Source: CAD feature listing. Evaluate the final solid. Frame: model axes, mm. Face numbers are marked on the shaded views. Give positions to 0.01 mm unless a question says otherwise; leave off trailing zeros. Order: outer loops, then holes, each group sorted by start corner. A loop starts at its lowest first (then second) coordinate and runs counter-clockwise, first axis right, second up.
1) Draft query along X for the marked faces 1, 2 and 3. Return one class per face: released by +X, released by -X, zero draft, split by the parting line, or undercut.
2) First-contact query: P1, Ø3, axis at x = -108.5, y = 10.5, coming from the -Z side; P2, Ø5, axis at x = -142, z = 5, coming from the +Y side. Flat tips, straight axial feed; report the tip coordinate or a pass-through.
3) Material intervals for line 1 (X direction, y = 13.5, z = -7.75); line 2 (X direction, y = 14.75, z = 5.5); line 3 (Z direction, x = 1.35, y = 10), sorted ascending.
4) Section A-A, the plane x = -133. Return loops of the section in (y, z), plus the area to 3 significant figures.
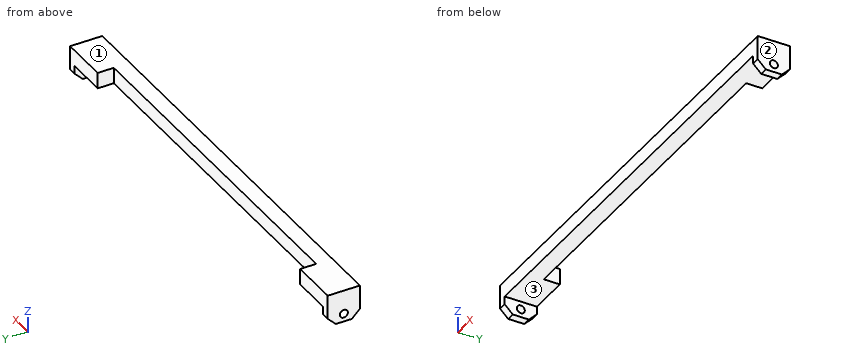
Autodesk Fusion 360 part; units mm, degrees
sketch "Sketch1" plane through (0, 0, 0) normal (0, 1, 0) x (1, 0, 0)
  line L0 (0, 0) -> (-25, 0)
  line L1 (-25, 0) -> (-25, -5)
  line L2 (-25, -5) -> (5, -5)
  line L3 (0, 0) -> (0, 10)
  line L4 (0, 10) -> (5, 10)
  line L5 (5, 10) -> (5, -5)
  line L6 (-25, 0) -> (-245, 0)
  line L7 (-245, 0) -> (-245, -5)
  line L8 (-245, -5) -> (-25, -5)
  line L9 (-25, 0) -> (-140, 0)
  line L10 (-140, 0) -> (-140, 27.0089)
  line L11 (-270, 10) -> (-275, 10)
  line L12 (-270, 0) -> (-270, 10)
  line L13 (-275, 10) -> (-275, -5)
  line L14 (-270, 0) -> (-245, 0)
  line L15 (-245, -5) -> (-275, -5)
  line L16 (-245, 0) -> (-245, -5)
  point P0 (-270, 0)
  dimension "d1" = 25
  dimension "d2" = 5
  dimension "d3" = 30
  dimension "d4" = 10
  dimension "d5" = 5
  dimension "d6" = 220
  dimension "d7" = 5
  dimension "d8" = 115
extrude "Extrude1" add sketch "Sketch1" along normal blind 10
extrude "Extrude2" add sketch "Sketch1" along normal blind 20 contours L0 L1 L2 L3 L4 L5 | L7 L11 L12 L13 L14 L15 L16
sketch "Sketch2" plane through (5, 0, 0) normal (1, 0, 0) x (0, 0, -1)
  line L0 (-5, 0) -> (10, 0)
  line L1 (10, 0) -> (10, 20)
  line L2 (10, 20) -> (-5, 20)
  line L3 (-5, 20) -> (-5, 0)
sketch "Sketch3" plane through (0, 0, 0) normal (-1, 0, 0) x (0, 0, 1)
  line L0 (-10, 0) -> (0, 0)
  line L1 (0, 0) -> (0, 20)
  line L2 (0, 20) -> (-10, 20)
  line L3 (-10, 20) -> (-10, 0)
  line L4 (-10, 0) -> (-5, 0)
  line L5 (-5, 0) -> (-5, 10)
  circle A0 centre (-5, 10) radius 2.5
  dimension "d13" = 5
  dimension "d14" = 10
  dimension "d15" = 5
extrude "Extrude3" cut sketch "Sketch3" along normal mid plane 662 contours A0
chamfer "Chamfer1" distance 5 angle 45 4 edges at (2.5, 20, -10) (2.5, 0, -10) (-272.5, 20, -10) (-272.5, 0, -10)
sketch "Sketch5" plane through (0, 10, 0) normal (0, 1, 0) x (-1, 0, 0)
  line L0 (25, 5) -> (25, 0)
  line L1 (25, 0) -> (245, 0)
  line L2 (245, 0) -> (245, 5)
  line L3 (245, 5) -> (25, 5)
  line L4 (245, 0) -> (135, 0)
  dimension "d30" = 110
sketch "Sketch6" plane through (0, 0, 5) normal (0, 0, 1) x (1, 0, 0)
  line L0 (-25, 10) -> (-245, 10)
  line L1 (-245, 10) -> (-245, 20)
  line L2 (-245, 20) -> (-275, 20)
  line L3 (-275, 20) -> (-275, 0)
  line L4 (-275, 0) -> (5, 0)
  line L5 (5, 0) -> (5, 20)
  line L6 (5, 20) -> (-25, 20)
  line L7 (-25, 20) -> (-25, 10)
extrude "Extrude5" add 1 faces at (-265, 10, 5) along direction (0, 0, 1) blind 5
sketch "Sketch7" plane through (0, 10, 0) normal (0, 1, 0) x (-1, 0, 0)
  line L0 (25, 10) -> (25, 0)
  line L1 (25, 0) -> (245, 0)
  line L2 (245, 0) -> (245, 10)
  line L3 (245, 10) -> (25, 10)
  line L4 (245, 0) -> (135, 0)
  line L5 (138.2622, 1.9923) -> (132.3533, 3.0342)
  line L6 (138.2622, 7.9923) -> (132.3533, 6.9504)
  line L7 (132.3533, 3.0342) -> (132.3533, 0)
  line L8 (138.2622, 7.9923) -> (138.2622, 1.9923)
  line L9 (132.3533, 6.9504) -> (132.3533, 10)
  line L10 (138.2622, 1.9923) -> (141.0619, 1.9923) construction
  line L11 (138.2622, 7.9923) -> (141.0619, 7.9923) construction
  line L12 (25, 0) -> (245, 0)
  line L13 (128.521, 0) -> (128.521, 5)
  line L14 (270, -5) -> (275, -5)
  line L15 (275, -5) -> (275, 10)
  line L16 (275, 10) -> (245, 10)
  line L17 (245, 10) -> (245, 0)
  line L18 (245, 0) -> (270, 0)
  line L19 (270, 0) -> (270, -5)
  point P0 (132.1074, 10.0354)
  point P1 (138.2622, 4.9923)
  dimension "d33" = 110
  dimension "d34" = 6
  dimension "d35" = 170
  dimension "d36" = 6
  dimension "d37" = 170
  dimension "d38" = 6
  dimension "d41" = 5
From the geometry:
1. face 1: zero draft
1. face 2: released by +X
1. face 3: undercut
2. P1: stops at z = 0
2. P2: stops at y = 10
3. line 1: x = -275 to -270, 0 to 5
3. line 2: x = -275 to -245, -25 to 5
3. line 3: z = -10 to -7.5, -2.5 to 10
4. outline: (0, 0) - (10, 0) - (10, 10) - (0, 10) - close
4. area: 100 mm2
